from build123d import *

# Parameters (mm, degrees)
CROQUIS1_R              = 2.5
SALIENTE_EXTRUIR1_DEPTH = 2
CROQUIS2_W              = 100
CROQUIS2_H              = 100
CORTAR_EXTRUIR1_DEPTH   = 10


with BuildPart() as part:
    # Croquis1 → Saliente-Extruir1 (new body)
    with BuildSketch(Plane(origin=(0, 0, 0), x_dir=(1, 0, 0), z_dir=(0, 1, 0))):
        with BuildLine():
            Line((17.5, 10), (157.5, 10))
            ThreePointArc((157.5, 10), (162.803300859, 12.196699141), (165, 17.5))
            Line((165, 17.5), (165, 157.5))
            ThreePointArc((165, 157.5), (162.803300859, 162.803300859), (157.5, 165))
            Line((157.5, 165), (17.5, 165))
            ThreePointArc((17.5, 165), (12.196699141, 162.803300859), (10, 157.5))
            Line((10, 157.5), (10, 17.5))
            ThreePointArc((10, 17.5), (12.196699141, 12.196699141), (17.5, 10))
        make_face()
        with Locations(Location((17.5, 157.5, 0), (0, 0, 270))):
            Circle(CROQUIS1_R, mode=Mode.SUBTRACT)
        with Locations(Location((157.5, 157.5, 0), (0, 0, 270))):
            Circle(CROQUIS1_R, mode=Mode.SUBTRACT)
        with Locations(Location((157.5, 17.5, 0), (0, 0, 270))):
            Circle(CROQUIS1_R, mode=Mode.SUBTRACT)
        with Locations(Location((17.5, 17.5, 0), (0, 0, 270))):
            Circle(CROQUIS1_R, mode=Mode.SUBTRACT)
    extrude(amount=SALIENTE_EXTRUIR1_DEPTH)

    # Croquis2 → Cortar-Extruir1 (cut)
    with BuildSketch(Plane(origin=(0, 2, 0), x_dir=(1, 0, 0), z_dir=(0, 1, 0))):
        with Locations((87.5, 87.5)):
            Rectangle(CROQUIS2_W, CROQUIS2_H)
    extrude(amount=-CORTAR_EXTRUIR1_DEPTH, mode=Mode.SUBTRACT)


solid = part.part
Verification items for the finished model (mm, model axes). Give positions to 0.01 mm unless a question says otherwise; leave off trailing zeros. Loops run counter-clockwise (first coordinate to the right, second up) from the corner with the lowest first, then second, coordinate; pieces in that order, holes last. Notation, with made-up numbers: (65.25, 53.25) - (95.25, 53.25) arc R38 cw to (95.25, 92.25) - close; hole circle Ø3 at (68.25, 50). An arc over 180 degrees is marked (long way). Write item = value, one per line. Start each with the question number.
Q1. Cross-section at A-A, the plane x = 103.5. Enter the section's corners in (y, z), and give its area (3 significant figures).
Q2. Cross-section at C-C, the plane z = -87.5. Enter the section's corners in (x, y).
Q3. Thickness scan on line 1 (X direction, y = 1.35, z = -17.5); line 2 (Z direction, x = 157.5, y = 1.65); line 3 (Z direction, x = 49, y = 0.45). Record the ranges inside material, lowest first.
Q4. Mould release check, pull along X, two halves, no side actions. Record for faces 1 (the face through (86, 0, -37)), 2 (the face through (18.251, 0.986, -155.115)), 3 (the face through (12.139, 0.986, -12.255)): released by +X, released by -X, zero draft, split by the parting line, or undercut.
Q5. Cross-section at B-B, the plane y = 1.5. Enter the section's corners in (x, z).
Answer key:
q1.outline = (0, -165) - (2, -165) - (2, -137.5) - (0, -137.5) - close; (0, -37.5) - (2, -37.5) - (2, -10) - (0, -10) - close
q1.area = 110 mm^2
q2.outline = (10, 0) - (37.5, 0) - (37.5, 2) - (10, 2) - close; (137.5, 0) - (165, 0) - (165, 2) - (137.5, 2) - close
q3.line_1 = 10 to 15, 20 to 155, 160 to 165
q3.line_2 = -165 to -160, -155 to -20, -15 to -10
q3.line_3 = -165 to -137.5, -37.5 to -10
q4.face_1 = zero draft
q4.face_2 = undercut
q4.face_3 = released by -X
q5.outline = (10, -157.5) arc R7.5 ccw to (17.5, -165) - (157.5, -165) arc R7.5 ccw to (165, -157.5) - (165, -17.5) arc R7.5 ccw to (157.5, -10) - (17.5, -10) arc R7.5 ccw to (10, -17.5) - close; hole circle Ø5 at (17.5, -157.5); hole circle Ø5 at (17.5, -17.5); hole (37.5, -137.5) - (137.5, -137.5) - (137.5, -37.5) - (37.5, -37.5) - close; hole circle Ø5 at (157.5, -157.5); hole circle Ø5 at (157.5, -17.5)
